Work out the finished part from the listing and answer in its coordinate system (mm). Face numbers are marked on the shaded views. A direction names the side the tool comes from. Coordinates: 2 decimals unless noted, no trailing zeros. Order: outer loops, then holes, each group sorted by start corner. A loop starts at its lowest first (then second) coordinate and runs counter-clockwise, first axis right, second up. Notation, with made-up numbers: (5, -33) - (25, -33) arc R21 cw to (25, -19) - close; hole circle Ø10 at (8, 28). An arc over 180 degrees is marked (long way). Answer as a JSON object with one key per item and string values. Group by question number.
1) The mould has two halves that part along Y. Classify the marked faces 1, 2 and 3: released by +Y, released by -Y, zero draft, split by the parting line, or undercut.
2) Section B-B (y = 70) is taken. Give the vertices of the cut face in (x, z), plus the area to 3 significant figures.
3) Section A-A (x = -9) is taken. Give the vertices of the cut face in (y, z).
4) Each of these flat-tipped pins is pushed along its axis until it touches: P1, Ø18, axis at y = 21, z = 22, coming from the -X side; P2, Ø0.5, axis at x = -17, z = 26.5, coming from the -Y side; P3, Ø8, axis at x = -15.5, z = 29, coming from the +Y side. Where does it stop, or does it pass through?
5) A tool of negligible diameter and unlimited length cuts with its end or side. For the marked faces 4, 5, 6 and 7, from which of +Z, -Z, +X, -X, +Y, -Y can it reach the whole face along a straight path? Write none if from no direction.
6) Find the intervals of material crossed by line 1 along Y through (x, z) = (7, 12.5); line 2 along Y through (x, z) = (1, 34); line 3 along Y through (x, z) = (-1, 26), in increasing order.
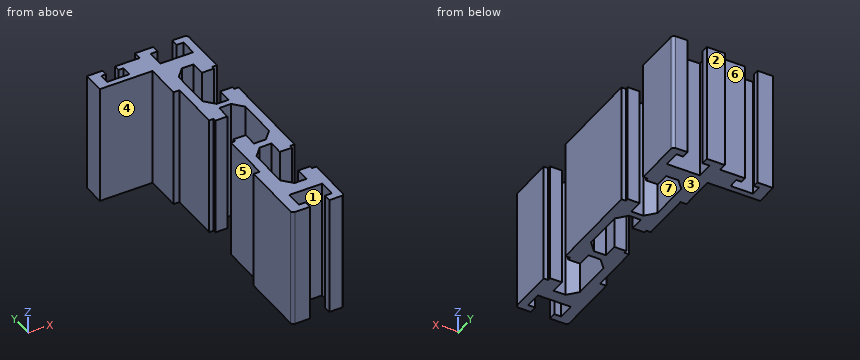
from build123d import *

# Parameters (mm, degrees)
EXTRUDE_1_DEPTH = 40


with BuildPart() as part:
    # Model → Бобышка-Вытянуть1 (new body)
    with BuildSketch(Plane.XY):
        with BuildLine():
            Line((-2.7, -8), (2.3, -8))
            Line((2.3, -8), (2.3, -5.5))
            Line((2.3, -5.5), (0, -5.5))
            Line((0, -5.5), (0, 0))
            Line((0, 0), (11, 0))
            Line((11, 0), (11, -5.5))
            Line((11, -5.5), (8.7, -5.5))
            Line((8.7, -5.5), (8.7, -8))
            Line((8.7, -8), (12.7, -8))
            ThreePointArc((12.7, -8), (13.407106781, -7.707106781), (13.7, -7))
            Line((13.7, -7), (13.7, 8))
            Line((13.7, 8), (12.2, 8))
            Line((12.2, 8), (12.2, 9))
            Line((12.2, 9), (8.2, 9))
            Line((8.2, 9), (8.2, 4.25))
            Line((8.2, 4.25), (4.2, 4.25))
            Line((4.2, 4.25), (1.3, 7.5))
            Line((1.3, 7.5), (1.3, 21))
            Line((1.3, 21), (4.2, 24.25))
            Line((4.2, 24.25), (8.2, 24.25))
            Line((8.2, 24.25), (8.2, 19.5))
            Line((8.2, 19.5), (12.2, 19.5))
            Line((12.2, 19.5), (12.2, 20.5))
            Line((12.2, 20.5), (13.7, 20.5))
            Line((13.7, 20.5), (13.7, 52.6))
            Line((13.7, 52.6), (12.2, 52.6))
            Line((12.2, 52.6), (12.2, 53.6))
            Line((12.2, 53.6), (8.2, 53.6))
            Line((8.2, 53.6), (8.2, 48.85))
            Line((8.2, 48.85), (4.2, 48.85))
            Line((4.2, 48.85), (1.3, 52.1))
            Line((1.3, 52.1), (1.3, 65.6))
            Line((1.3, 65.6), (4.2, 68.85))
            Line((4.2, 68.85), (8.2, 68.85))
            Line((8.2, 68.85), (8.2, 64.1))
            Line((8.2, 64.1), (12.2, 64.1))
            Line((12.2, 64.1), (12.2, 65.1))
            Line((12.2, 65.1), (13.7, 65.1))
            Line((13.7, 65.1), (13.7, 81))
            ThreePointArc((13.7, 81), (13.407106781, 81.707106781), (12.7, 82))
            Line((12.7, 82), (8.7, 82))
            Line((8.7, 82), (8.7, 79.5))
            Line((8.7, 79.5), (11, 79.5))
            Line((11, 79.5), (11, 74))
            Line((11, 74), (0, 74))
            Line((0, 74), (0, 79.5))
            Line((0, 79.5), (2.3, 79.5))
            Line((2.3, 79.5), (2.3, 82))
            Line((2.3, 82), (-3.7, 82))
            Line((-3.7, 82), (-3.7, 79.35))
            Line((-3.7, 79.35), (-11.9, 79.35))
            Line((-11.9, 79.35), (-11.9, 77.35))
            Line((-11.9, 77.35), (-10.25, 77.35))
            Line((-10.25, 77.35), (-10.25, 74))
            Line((-10.25, 74), (-17.75, 74))
            Line((-17.75, 74), (-17.75, 77.35))
            Line((-17.75, 77.35), (-16.1, 77.35))
            Line((-16.1, 77.35), (-16.1, 79.35))
            Line((-16.1, 79.35), (-21.3, 79.35))
            Line((-21.3, 79.35), (-21.3, 72))
            Line((-21.3, 72), (-3.7, 72))
            Line((-3.7, 72), (-3.7, 60))
            Line((-3.7, 60), (-1.7, 60))
            Line((-1.7, 60), (-1.7, 43))
            Line((-1.7, 43), (-0.2, 43))
            Line((-0.2, 43), (-0.2, 42))
            Line((-0.2, 42), (3.8, 42))
            Line((3.8, 42), (3.8, 46.75))
            Line((3.8, 46.75), (7.8, 46.75))
            Line((7.8, 46.75), (10.7, 43.5))
            Line((10.7, 43.5), (10.7, 30))
            Line((10.7, 30), (7.8, 26.75))
            Line((7.8, 26.75), (3.8, 26.75))
            Line((3.8, 26.75), (3.8, 31.5))
            Line((3.8, 31.5), (-0.2, 31.5))
            Line((-0.2, 31.5), (-0.2, 30.5))
            Line((-0.2, 30.5), (-1.7, 30.5))
            Line((-1.7, 30.5), (-1.7, 14))
            Line((-1.7, 14), (-3.7, 14))
            Line((-3.7, 14), (-3.7, -7))
            ThreePointArc((-3.7, -7), (-3.407106781, -7.707106781), (-2.7, -8))
        make_face()
    extrude(amount=EXTRUDE_1_DEPTH)


solid = part.part
Report:
{
 "1": {"face 1": "undercut", "face 2": "released by +Y", "face 3": "zero draft"},
 "2": {"outline": "(-3.7, 0) - (13.7, 0) - (13.7, 40) - (-3.7, 40) - close", "area": "696 mm²"},
 "3": {"outline": "(72, 0) - (79.35, 0) - (79.35, 40) - (72, 40) - close"},
 "4": {"P1": "stops at x = -3.7", "P2": "stops at y = 72", "P3": "stops at y = 79.35"},
 "5": {"face 4": "+Z, -Z, -X, -Y", "face 5": "+Z, -Z, -X", "face 6": "+Z, -Z, -X, +Y", "face 7": "+Z, -Z"},
 "6": {"line 1": "y = 0 to 4.25, 24.25 to 26.75, 46.75 to 48.85, 68.85 to 74", "line 2": "y = -8 to -5.5, 0 to 31.5, 42 to 74, 79.5 to 82", "line 3": "y = -8 to 30.5, 43 to 82"}
}
